Model file for the job. Use its own axes, mm. Face numbers are marked on the shaded views. A direction names the side the tool comes from. Coordinates: 2 decimals unless noted, no trailing zeros. Loops run counter-clockwise (first coordinate to the right, second up) from the corner with the lowest first, then second, coordinate; pieces in that order, holes last.
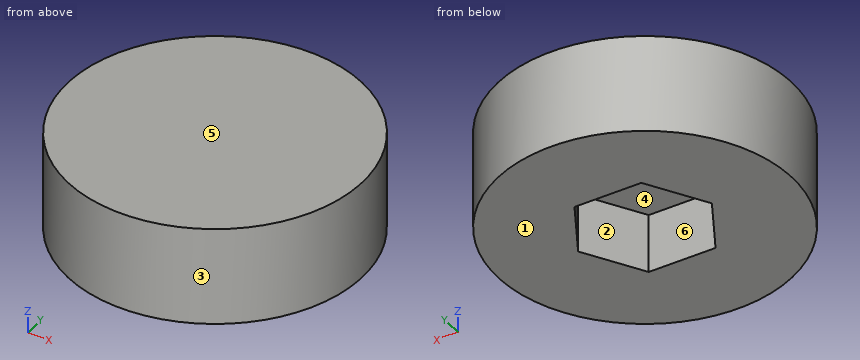
Autodesk Inventor part; units mm, degrees
ref_plane "YZ Plane" through (0, 0, 0) normal (1, 0, 0) x (0, 1, 0)
ref_plane "XZ Plane" through (0, 0, 0) normal (0, 1, 0) x (-1, 0, 0)
ref_plane "XY Plane" through (0, 0, 0) normal (0, 0, 1) x (1, 0, 0)
sketch "Эскиз1" plane through (0, 0, 0) normal (0, 0, 1) x (1, 0, 0)
  circle A0 centre (0, 0) radius 7.5
  dimension "d0" = 15
extrude "Выдавливание1" add sketch "Эскиз1" along normal blind 5
sketch "Эскиз2" plane through (0, 0, 0) normal (0, 0, -1) x (-1, 0, 0)
  circle A0 centre (0, 0) radius 3 construction
  line L0 (1.7321, 3) -> (3.4641, 0)
  line L1 (3.4641, 0) -> (1.7321, -3)
  line L2 (1.7321, -3) -> (-1.7321, -3)
  line L3 (-1.7321, -3) -> (-3.4641, 0)
  line L4 (-3.4641, 0) -> (-1.7321, 3)
  line L5 (-1.7321, 3) -> (1.7321, 3)
  point P0 (0, 3)
  dimension "d3" = 6
extrude "Выдавливание2" cut sketch "Эскиз2" against normal blind 3
properties part number "hand"
Q1. Flat gauge pins, fed straight in: P1, Ø1.5, axis at y = -4.5, z = 3, coming from the +X side; P2, Ø1.5, axis at y = -2, z = 4.5, coming from the -X side; P3, Ø1.5, axis at y = -2.5, z = 4, coming from the +X side. Where does each tip first touch, or does it go through?
Answers:
P1: stops at x = 6.5
P2: stops at x = -7.4
P3: stops at x = 7.29
Q2. Which spindle directions (+Z, -Z, +X, -X, +Y, -Y) get a long thin tool onto all of the face, cutting with end or side? Do the marked faces 5 and 6. Say none if no direction does.
Answers:
face 5: +Z, +X, -X, +Y, -Y
face 6: -Z
Q3. Drill centre lines: line 1 (X direction, y = -1, z = 2.2); line 2 (Y direction, x = 1.5, z = 1.65); line 3 (Y direction, x = 2, z = 1). Where is each one in solid material? Low to high.
Answers:
line 1: x = -7.43 to -2.89, 2.89 to 7.43
line 2: y = -7.35 to -3, 3 to 7.35
line 3: y = -7.23 to -2.54, 2.54 to 7.23
Q4. Slice it at D-D (x = 4.5). List the corners of the cut face in (y, z), and give its area (3 significant figures).
Answers:
outline: (-6, 0) - (6, 0) - (6, 5) - (-6, 5) - close
area: 60.0 mm2
Q5. Slice it at A-A (z = 2). List the corners of the cut face in (x, y), and give its area (3 significant figures).
Answers:
outline: circle Ø15 at (0, 0); hole (-3.46, 0) - (-1.73, -3) - (1.73, -3) - (3.46, 0) - (1.73, 3) - (-1.73, 3) - close
area: 146 mm2
Q6. Slice it at C-C (y = 1.25). List the corners of the cut face in (x, z).
Answers:
outline: (-7.4, 0) - (-2.74, 0) - (-2.74, 3) - (2.74, 3) - (2.74, 0) - (7.4, 0) - (7.4, 5) - (-7.4, 5) - close
Q7. Mould opens along Y. For the marked faces 1, 2, 3 and 4 say: +Y half, -Y half, draft (parallel to the pull), parting line (faces both ways), or undercut.
Answers:
face 1: draft
face 2: undercut
face 3: parting line
face 4: undercut
Q8. Slice it at B-B (x = 0). List the corners of the cut face in (y, z).
Answers:
outline: (-7.5, 0) - (-3, 0) - (-3, 3) - (3, 3) - (3, 0) - (7.5, 0) - (7.5, 5) - (-7.5, 5) - close
